Geometry: see drawing. Coordinates: mm, zero at the bounding-box minimum. A direction names the side the tool comes from. Coordinates: 2 decimals unless noted, no trailing zeros. Order: outer loops, then holes, each group sorted by start corner. A loop starts at its lowest first (then second) coordinate and runs counter-clockwise, first axis right, second up. Notation, with made-up numbers: M 67,85 L 79,85 A12 ccw 79,91 Z; hole C 29.5,-36.5 d3. An arc over 180 degrees is marked long. Answer in a Markdown table with one row per item.
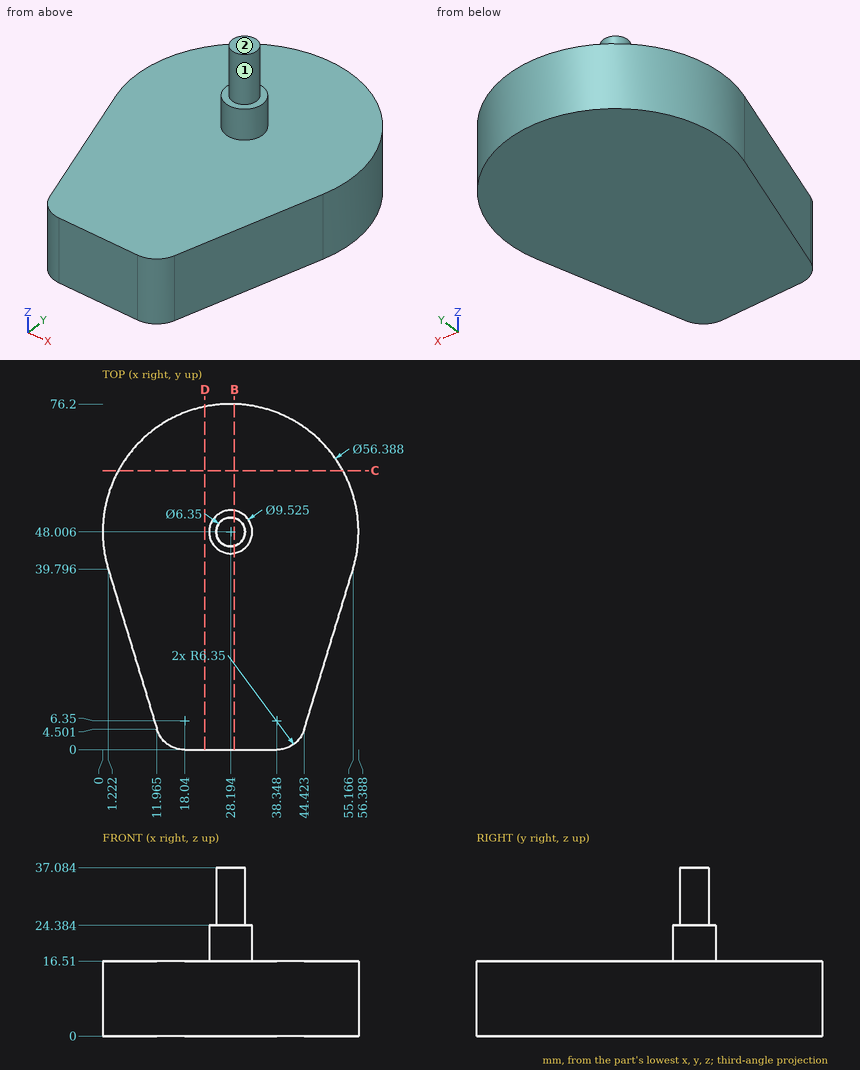
1) Cut plane C-C, the plane y = 61.5. Output: boundary loops of the cut face in (x, z).
Resolved:
| item | result |
|---|---|
| outline | M 3.44,0 L 52.95,0 L 52.95,16.51 L 3.44,16.51 Z |
2) Material intervals for probe 1 along Z at (x, y) = (39, 37); probe 2 along X at (y, z) = (48, 18.5); probe 3 along Y at (x, z) = (30, 20.5), sorted ascending.
Resolved:
| item | result |
|---|---|
| probe 1 | z = 0 to 16.51 |
| probe 2 | x = 23.43 to 32.96 |
| probe 3 | y = 43.6 to 52.41 |
3) Cut plane B-B, the plane x = 29. Output: boundary loops of the cut face in (y, z) (1 decimal), and give its area (3 significant figures).
Resolved:
| item | result |
|---|---|
| outline | M 0,0 L 76.2,0 L 76.2,16.5 L 52.7,16.5 L 52.7,24.4 L 51.1,24.4 L 51.1,37.1 L 44.9,37.1 L 44.9,24.4 L 43.3,24.4 L 43.3,16.5 L 0,16.5 Z |
| area | 1,410 mm2 |
4) Contact query for flat-ended pins moving along their axis: pin 1 (3 mm diameter, centred on y = 55, z = 12.5, fed in from -X); pin 2 (1 mm diameter, centred on x = 18.5, z = 12.5, fed in from +Y); pin 3 (12 mm diameter, centred on x = 33.5, z = 11, fed in from +Y). Output: stop coordinate, or through.
Resolved:
| item | result |
|---|---|
| pin 1 | stops at x = 0.54 |
| pin 2 | stops at y = 74.66 |
| pin 3 | stops at y = 76.2 |
5) Reachability of the marked faces 1 and 2 from +Z, -Z, +X, -X, +Y, -Y: full face, straight path, thin tool, end or side. Return the list, or none.
Resolved:
| item | result |
|---|---|
| face 1 | +Z |
| face 2 | +Z, +X, -X, +Y, -Y |
6) Cut plane D-D, the plane x = 22.5. Output: boundary loops of the cut face in (y, z), and give its area (3 significant figures).
Resolved:
| item | result |
|---|---|
| outline | M 0,0 L 75.62,0 L 75.62,16.51 L 0,16.51 Z |
| area | 1,250 mm2 |
